from build123d import *

# Parameters (mm, degrees)
BOSS_EXTRUDE1_DEPTH = 558.8
CUT_EXTRUDE1_REACH  = 5.175
SKETCH2_R           = 2.54


with BuildPart() as part:
    # Sketch1 → Boss-Extrude1 (new body)
    with BuildSketch(Plane(origin=(0, 0, 0), x_dir=(0, 0, -1), z_dir=(1, 0, 0))):
        Polygon((3.175, 3.175), (3.175, 19.05), (0, 19.05), (0, 0), (19.05, 0), (19.05, 3.175), align=None)
    extrude(amount=BOSS_EXTRUDE1_DEPTH)

    # Sketch2 → Cut-Extrude1 (cut, up to next)
    with BuildSketch(Plane(origin=(0, 3.175, 0), x_dir=(1, 0, 0), z_dir=(0, 1, 0)), mode=Mode.PRIVATE) as cut_extrude1_sk1:
        with Locations((552.45, 11.1125)):
            Circle(SKETCH2_R)
    cut_extrude1_tool1 = extrude(cut_extrude1_sk1.sketch, amount=-CUT_EXTRUDE1_REACH, mode=Mode.PRIVATE) & part.part
    add(cut_extrude1_tool1.solids().sort_by_distance((552.45, 3.175, -11.1125))[0], mode=Mode.SUBTRACT)
    # Sketch2 → Cut-Extrude1 (cut, up to next)
    with BuildSketch(Plane(origin=(0, 3.175, 0), x_dir=(1, 0, 0), z_dir=(0, 1, 0)), mode=Mode.PRIVATE) as cut_extrude1_sk2:
        with Locations((6.35, 11.1125)):
            Circle(SKETCH2_R)
    cut_extrude1_tool2 = extrude(cut_extrude1_sk2.sketch, amount=-CUT_EXTRUDE1_REACH, mode=Mode.PRIVATE) & part.part
    add(cut_extrude1_tool2.solids().sort_by_distance((6.35, 3.175, -11.1125))[0], mode=Mode.SUBTRACT)


solid = part.part
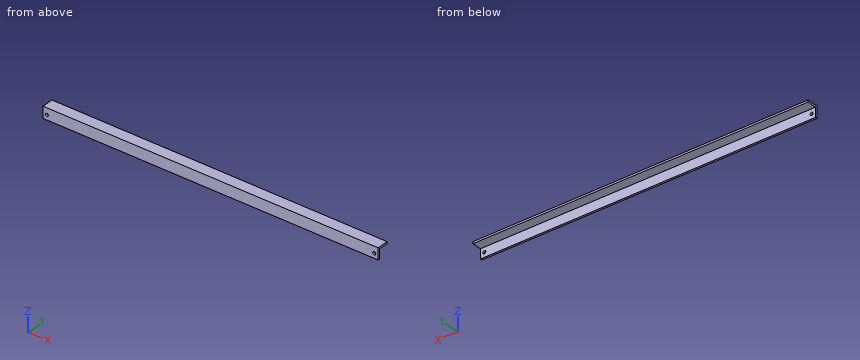
Geometry: final body of the model. Coordinates: model frame, mm. Coordinates: 2 decimals unless noted, no trailing zeros. Order: outer loops, then holes, each group sorted by start corner. A loop starts at its lowest first (then second) coordinate and runs counter-clockwise, first axis right, second up.
(1) Section query A-A (y = 11). Return the cut outline in (x, z) (3 decimals), plus the area to 3 significant figures.
(2) First-contact query: pin 1 (8 mm diameter, centred on y = 4, z = -6.5, fed in from +X); pin 2 (6 mm diameter, centred on x = 372.5, z = -13, fed in from +Y) (3 decimals); pin 3 (5 mm diameter, centred on x = 275, y = 9, fed in from -Z) (3 decimals). Flat tips, straight axial feed; report the tip coordinate or a pass-through.
(3) Section query B-B (x = 63). Return the cut outline in (y, z) (3 decimals).
(4) Material intervals for probe 1 along Z at (x, y) = (552.45, 1.9); probe 2 along Z at (x, y) = (391, 13) (3 decimals); probe 3 along Y at (x, z) = (84, -11) (3 decimals), sorted ascending.
Solution:
1. outline: (0, -3.175) - (558.8, -3.175) - (558.8, 0) - (0, 0) - close
1. area: 1,770 mm2
2. pin 1: stops at x = 558.8
2. pin 2: stops at y = 3.175
2. pin 3: stops at z = -3.175
3. outline: (0, -19.05) - (3.175, -19.05) - (3.175, -3.175) - (19.05, -3.175) - (19.05, 0) - (0, 0) - close
4. probe 1: z = -19.05 to -13.65, -8.57 to 0
4. probe 2: z = -3.175 to 0
4. probe 3: y = 0 to 3.175
